Answer from the drawing. Dimensions are ordinates in mm from the lowest x, y and z of the part. A direction names the side the tool comes from. Give positions to 0.01 mm unless a question says otherwise; leave off trailing zeros. Loops run counter-clockwise (first coordinate to the right, second up) from the corner with the lowest first, then second, coordinate; pieces in that order, holes last. Notation, with made-up numbers: (-26.5, 33.5) - (-19.5, 33.5) arc R14 cw to (-19.5, 42.5) - close; hole circle Ø10 at (-27.75, 38). An arc over 180 degrees is marked (long way). Write each question's results on one line, items separated by ' | '. Start each with the question number.
Q1. Find the intervals of material crossed by line 1 (X direction, y = 40, z = 21); line 2 (Z direction, x = 51.5, y = 41.5), in increasing order. Write a range as from..to.
Q2. The part is cut by section B-B, the plane x = 40. Write down the section's boundary in (y, z).
Q3. The part is cut by section C-C, the plane y = 40. Write down the section's boundary in (x, z), plus the area to 3 significant figures.
Q4. The part is cut by section A-A, the plane z = 19.5. Write down the section's boundary in (x, y) (1 decimal).
Q5. Determine the mould class of the marked faces 1, 2 and 3 for opening direction X: +X half, -X half, draft (parallel to the pull), parting line (faces both ways), or undercut.
Q6. For the marked faces 4, 5, 6, 7 and 8, determine the directions among +Z, -Z, +X, -X, +Y, -Y from which every point of the face is accessible in a straight line to the end or side of a thin tool.
Q7. The part is cut by section D-D, the plane x = 13. Write down the section's boundary in (y, z).
Q8. Given pin 1 (10 mm diameter, centred on x = 58.5, z = 24.5, fed in from -Y); pin 2 (18 mm diameter, centred on x = 49.5, y = 27, fed in from +Z); pin 3 (8 mm diameter, centred on y = 72, z = 24.5, fed in from +X) (1 decimal), each flat-ended and moving along its own axis, determine where each tip first touches the part or whether it passes through.
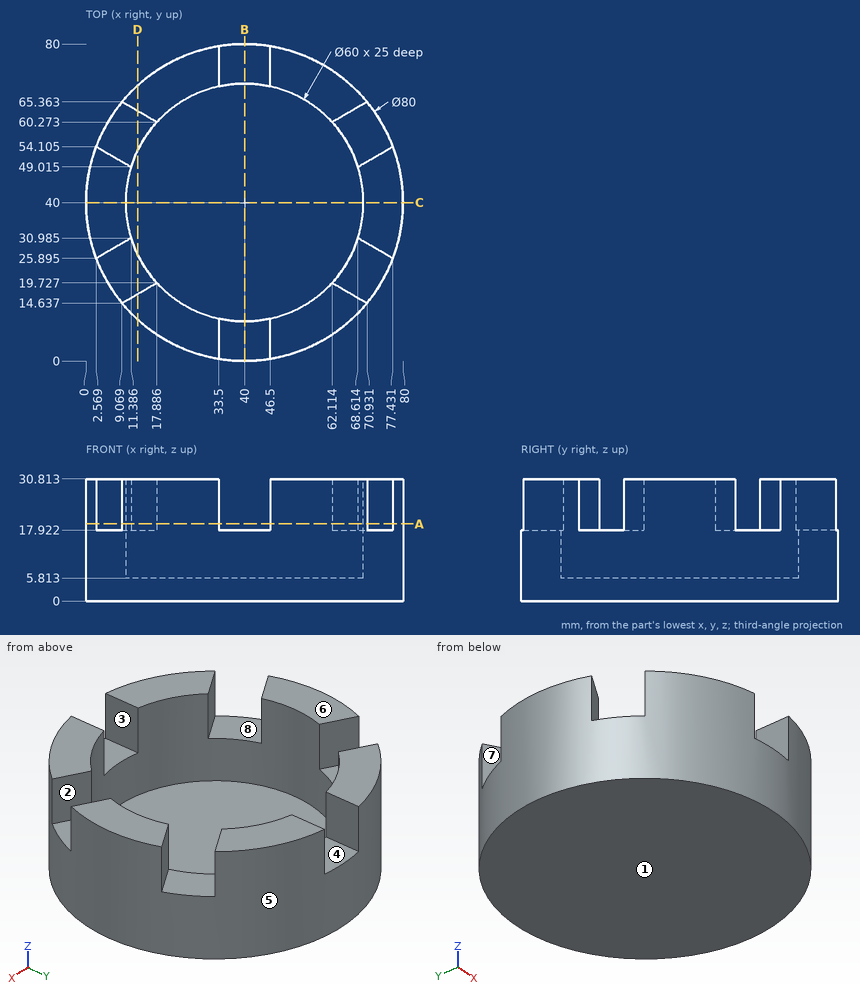
Check sheet entries:
1) line 1: x = 0..10, 70..80 | line 2: z = 0..5.81
2) outline: (0, 0) - (80, 0) - (80, 17.92) - (70, 17.92) - (70, 5.81) - (10, 5.81) - (10, 17.92) - (0, 17.92) - close
3) outline: (0, 0) - (80, 0) - (80, 30.81) - (70, 30.81) - (70, 5.81) - (10, 5.81) - (10, 30.81) - (0, 30.81) - close | area: 965 mm^2
4) outline: (2.6, 25.9) - (11.4, 31) arc R30 cw to (11.4, 49) - (2.6, 54.1) arc R40 ccw to start; (9.1, 14.6) arc R40 ccw to (33.5, 0.5) - (33.5, 10.7) arc R30 cw to (17.9, 19.7) - close; (9.1, 65.4) - (17.9, 60.3) arc R30 cw to (33.5, 69.3) - (33.5, 79.5) arc R40 ccw to start; (46.5, 0.5) arc R40 ccw to (70.9, 14.6) - (62.1, 19.7) arc R30 cw to (46.5, 10.7) - close; (46.5, 69.3) arc R30 cw to (62.1, 60.3) - (70.9, 65.4) arc R40 ccw to (46.5, 79.5) - close; (68.6, 31) - (77.4, 25.9) arc R40 ccw to (77.4, 54.1) - (68.6, 49) arc R30 cw to start
5) face 1: draft | face 2: +X half | face 3: undercut
6) face 4: +Z, +Y, -Y | face 5: +Z, -Z | face 6: +Z, +X, -X, +Y, -Y | face 7: +Z, -X | face 8: +Z
7) outline: (10.49, 0) - (69.51, 0) - (69.51, 30.81) - (63.09, 30.81) - (63.09, 17.92) - (53.08, 17.92) - (53.08, 5.81) - (26.92, 5.81) - (26.92, 17.92) - (16.91, 17.92) - (16.91, 30.81) - (10.49, 30.81) - close
8) pin 1: stops at y = 2.35 | pin 2: stops at z = 5.81 | pin 3: stops at x = 68.6
